Geometry check sheet. Reference: the model listing, model coordinates, mm. Coordinates: 2 decimals unless noted, no trailing zeros. Write each loop counter-clockwise with the first axis right and the second up, starting at its lowest first coordinate (ties: lowest second). Pieces come first, ordered by that corner, then holes. Notation, with made-up numbers: (83.25, 19.25) -> (104.25, 19.25) arc R21 ccw to (104.25, 23.25) -> close; hole circle Ø2 at (77.25, 71). An arc over 180 degrees is marked (long way). Use a Markdown table: item, result.
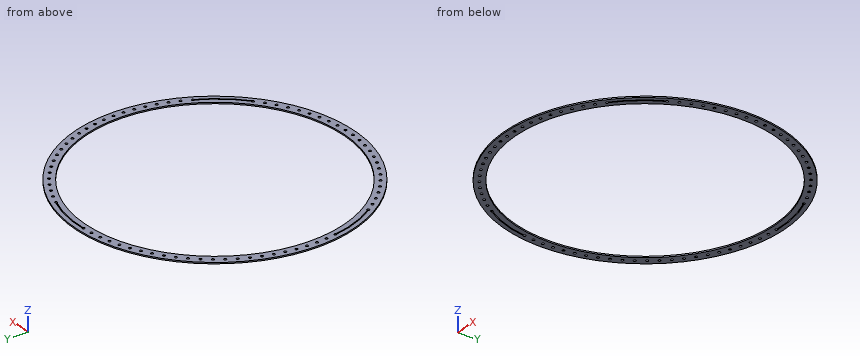
```python
from build123d import *

# Parameters (mm, degrees)
F0_R     = 685.8
F0_R_2   = 6.35
F0_R_3   = 635
F1_DEPTH = 6.35


with BuildPart() as f1:
    # F0 (on Top) → F1 (new body)
    with BuildSketch(Plane.XY):
        Circle(F0_R)
        with Locations((-352.110822, -558.700393)):
            Circle(F0_R_2, mode=Mode.SUBTRACT)
        with Locations((-393.085485, -530.671237)):
            Circle(F0_R_2, mode=Mode.SUBTRACT)
        with Locations((-532.658582, -390.388261)):
            Circle(F0_R_2, mode=Mode.SUBTRACT)
        with Locations((-431.838824, -499.643263)):
            Circle(F0_R_2, mode=Mode.SUBTRACT)
        with Locations((-501.827608, -429.298511)):
            Circle(F0_R_2, mode=Mode.SUBTRACT)
        with Locations((-468.16081, -465.782799)):
            Circle(F0_R_2, mode=Mode.SUBTRACT)
        with Locations((-264.434964, -605.146519)):
            Circle(F0_R_2, mode=Mode.SUBTRACT)
        with Locations((-218.229223, -623.301024)):
            Circle(F0_R_2, mode=Mode.SUBTRACT)
        with Locations((-309.146385, -583.572337)):
            Circle(F0_R_2, mode=Mode.SUBTRACT)
        with Locations((-122.386184, -648.96054)):
            Circle(F0_R_2, mode=Mode.SUBTRACT)
        with Locations((-170.79027, -637.933259)):
            Circle(F0_R_2, mode=Mode.SUBTRACT)
        with Locations((-73.290494, -656.320549)):
            Circle(F0_R_2, mode=Mode.SUBTRACT)
        with Locations((-23.78064, -659.971697)):
            Circle(F0_R_2, mode=Mode.SUBTRACT)
        with BuildLine():
            ThreePointArc((-561.930553, -343.089944), (-556.535629, -344.295153), (-554.129507, -349.271931))
            ThreePointArc((-554.129507, -349.271931), (-562.262715, -355.36641), (-565.827987, -345.849027))
            Line((-565.827987, -345.849027), (-601.958696, -284.23674))
            Line((-601.958696, -284.23674), (-634.753594, -200.992062))
            Line((-634.753594, -200.992062), (-649.807483, -131.860068))
            ThreePointArc((-649.807483, -131.860068), (-652.263014, -120.699131), (-641.979851, -125.684382))
            ThreePointArc((-641.979851, -125.684382), (-642.840203, -128.875975), (-645.188124, -131.202719))
            Line((-645.188124, -131.202719), (-630.639189, -198.568385))
            Line((-630.639189, -198.568385), (-598.505303, -280.938769))
            Line((-598.505303, -280.938769), (-561.930553, -343.089944))
        make_face(mode=Mode.SUBTRACT)
        with Locations((-655.939404, -76.62675)):
            Circle(F0_R_2, mode=Mode.SUBTRACT)
        with Locations((-659.842248, -27.136101)):
            Circle(F0_R_2, mode=Mode.SUBTRACT)
        with Locations((25.863599, -659.893351)):
            Circle(F0_R_2, mode=Mode.SUBTRACT)
        with Locations((75.361682, -656.085952)):
            Circle(F0_R_2, mode=Mode.SUBTRACT)
        with Locations((124.433897, -648.571018)):
            Circle(F0_R_2, mode=Mode.SUBTRACT)
        with Locations((172.802937, -637.391014)):
            Circle(F0_R_2, mode=Mode.SUBTRACT)
        with Locations((220.195469, -622.609119)):
            Circle(F0_R_2, mode=Mode.SUBTRACT)
        with Locations((266.343678, -604.308866)):
            Circle(F0_R_2, mode=Mode.SUBTRACT)
        with Locations((310.986782, -582.593667)):
            Circle(F0_R_2, mode=Mode.SUBTRACT)
        with Locations((353.872502, -557.586238)):
            Circle(F0_R_2, mode=Mode.SUBTRACT)
        with Locations((394.758491, -529.427893)):
            Circle(F0_R_2, mode=Mode.SUBTRACT)
        with BuildLine():
            ThreePointArc((578.330809, -315.516767), (580.121908, -305.046288), (589.006867, -310.868357))
            ThreePointArc((589.006867, -310.868357), (587.146995, -315.358485), (582.656867, -317.218357))
            Line((582.656867, -317.218357), (547.185732, -379.019656))
            Line((547.185732, -379.019656), (491.732303, -449.04348))
            Line((491.732303, -449.04348), (439.763704, -498.277755))
            ThreePointArc((439.763704, -498.277755), (427.529669, -500.665355), (437.968229, -493.852961))
            Line((437.968229, -493.852961), (487.90386, -446.189437))
            Line((487.90386, -446.189437), (542.557285, -377.844919))
            Line((542.557285, -377.844919), (578.330809, -315.516767))
        make_face(mode=Mode.SUBTRACT)
        with Locations((604.36299, -266.220841)):
            Circle(F0_R_2, mode=Mode.SUBTRACT)
        with Locations((622.653864, -220.068912)):
            Circle(F0_R_2, mode=Mode.SUBTRACT)
        with Locations((637.361585, -172.911452)):
            Circle(F0_R_2, mode=Mode.SUBTRACT)
        with Locations((648.549823, -124.544316)):
            Circle(F0_R_2, mode=Mode.SUBTRACT)
        with Locations((656.073112, -75.473382)):
            Circle(F0_R_2, mode=Mode.SUBTRACT)
        with Locations((659.888938, -25.975947)):
            Circle(F0_R_2, mode=Mode.SUBTRACT)
        with Locations((-660.016329, 22.507894)):
            Circle(F0_R_2, mode=Mode.SUBTRACT)
        with Locations((-656.460664, 72.024697)):
            Circle(F0_R_2, mode=Mode.SUBTRACT)
        with Locations((-649.195345, 121.134488)):
            Circle(F0_R_2, mode=Mode.SUBTRACT)
        with Locations((-638.261428, 169.55975)):
            Circle(F0_R_2, mode=Mode.SUBTRACT)
        with Locations((-623.720702, 217.026832)):
            Circle(F0_R_2, mode=Mode.SUBTRACT)
        with Locations((-605.655336, 263.267496)):
            Circle(F0_R_2, mode=Mode.SUBTRACT)
        with Locations((-584.167416, 308.020438)):
            Circle(F0_R_2, mode=Mode.SUBTRACT)
        with Locations((-559.378371, 351.032759)):
            Circle(F0_R_2, mode=Mode.SUBTRACT)
        with Locations((-531.428284, 392.061398)):
            Circle(F0_R_2, mode=Mode.SUBTRACT)
        with Locations((-500.4751, 430.8745)):
            Circle(F0_R_2, mode=Mode.SUBTRACT)
        with Locations((-466.693735, 467.252734)):
            Circle(F0_R_2, mode=Mode.SUBTRACT)
        with Locations((-430.275088, 500.990527)):
            Circle(F0_R_2, mode=Mode.SUBTRACT)
        with Locations((-391.42496, 531.897227)):
            Circle(F0_R_2, mode=Mode.SUBTRACT)
        with Locations((-350.362894, 559.79818)):
            Circle(F0_R_2, mode=Mode.SUBTRACT)
        with Locations((-307.320929, 584.535719)):
            Circle(F0_R_2, mode=Mode.SUBTRACT)
        with Locations((-262.542296, 605.970051)):
            Circle(F0_R_2, mode=Mode.SUBTRACT)
        with Locations((-216.28004, 623.980051)):
            Circle(F0_R_2, mode=Mode.SUBTRACT)
        with Locations((-168.795586, 638.463946)):
            Circle(F0_R_2, mode=Mode.SUBTRACT)
        with Locations((-120.35727, 649.339886)):
            Circle(F0_R_2, mode=Mode.SUBTRACT)
        with Locations((-71.238816, 656.546412)):
            Circle(F0_R_2, mode=Mode.SUBTRACT)
        Circle(F0_R_3, mode=Mode.SUBTRACT)
        with Locations((659.975736, 23.668277)):
            Circle(F0_R_2, mode=Mode.SUBTRACT)
        with Locations((656.333018, 73.178752)):
            Circle(F0_R_2, mode=Mode.SUBTRACT)
        with Locations((648.981367, 122.275694)):
            Circle(F0_R_2, mode=Mode.SUBTRACT)
        with Locations((637.962328, 170.681658)):
            Circle(F0_R_2, mode=Mode.SUBTRACT)
        with Locations((623.338169, 218.1231)):
            Circle(F0_R_2, mode=Mode.SUBTRACT)
        with Locations((583.624962, 309.047025)):
            Circle(F0_R_2, mode=Mode.SUBTRACT)
        with Locations((605.191532, 264.331932)):
            Circle(F0_R_2, mode=Mode.SUBTRACT)
        with BuildLine():
            ThreePointArc((-15.43927, 659.09272), (-27.892825, 658.562438), (-16.552502, 663.736345))
            Line((-16.552502, 663.736345), (53.381546, 663.736345))
            Line((53.381546, 663.736345), (144.287124, 649.791609))
            Line((144.287124, 649.791609), (210.526942, 628.677552))
            ThreePointArc((210.526942, 628.677552), (217.501997, 630.270613), (221.532645, 624.359343))
            ThreePointArc((221.532645, 624.359343), (215.256126, 618.009768), (208.834346, 624.212392))
            Line((208.834346, 624.212392), (139.948994, 646.180678))
            Line((139.948994, 646.180678), (52.268314, 659.09272))
            Line((52.268314, 659.09272), (-15.43927, 659.09272))
        make_face(mode=Mode.SUBTRACT)
        with Locations((306.292743, 585.075136)):
            Circle(F0_R_2, mode=Mode.SUBTRACT)
        with Locations((261.476495, 606.430707)):
            Circle(F0_R_2, mode=Mode.SUBTRACT)
        with Locations((465.871506, 468.072537)):
            Circle(F0_R_2, mode=Mode.SUBTRACT)
        with Locations((499.716777, 431.753752)):
            Circle(F0_R_2, mode=Mode.SUBTRACT)
        with Locations((429.393599, 501.746248)):
            Circle(F0_R_2, mode=Mode.SUBTRACT)
        with Locations((558.760333, 352.015697)):
            Circle(F0_R_2, mode=Mode.SUBTRACT)
        with Locations((530.738153, 392.99513)):
            Circle(F0_R_2, mode=Mode.SUBTRACT)
        with Locations((390.489192, 532.584595)):
            Circle(F0_R_2, mode=Mode.SUBTRACT)
        with Locations((349.378134, 560.413311)):
            Circle(F0_R_2, mode=Mode.SUBTRACT)
    extrude(amount=F1_DEPTH)


solid = f1.part
```
Item 1: Depth check by flat-ended pin: P1, Ø3, axis at x = 408, z = 3.5, coming from the -Y side; P2, Ø1, axis at y = 294.5, z = 1.5, coming from the +X side; P3, Ø10, axis at x = -560.48, y = -349.27, coming from the -Z side; P4, Ø1, axis at x = 178, z = 1.5, coming from the -Y side. Enter the tip coordinate at first touch or a pass-through.
Answer block:
| item | result |
|---|---|
| P1 | stops at y = -552.34 |
| P2 | stops at x = 619.59 |
| P3 | passes through |
| P4 | stops at y = -662.43 |
Item 2: Section check B-B on z = 5. Count the separate pieces of the cut face and the enclosed holes in it, then the cut area to 3 significant figures.
Answer block:
| item | result |
|---|---|
| separate pieces | 1 |
| enclosed holes | 70 |
| area | 198,000 mm^2 |
Item 3: Section check A-A on y = 0. Record the boundary of the cut face in (x, z).
Answer block:
| item | result |
|---|---|
| outline | (-685.8, 0) -> (-635, 0) -> (-635, 6.35) -> (-685.8, 6.35) -> close; (635, 0) -> (685.8, 0) -> (685.8, 6.35) -> (635, 6.35) -> close |
Item 4: Thickness scan on L1, parallel to Y at x = 216.5, z = 6.25; L2, parallel to Y at x = 427, z = 3; L3, parallel to X at y = -176.5, z = 1.75. Record the ranges inside material, lowest first. Write a range as [from, to].
Answer block:
| item | result |
|---|---|
| L1 | y = [-650.73, -627.77], [-617.45, -596.95], [596.95, 618.15], [630.57, 650.73] |
| L2 | y = [-536.65, -470], [470, 495.86], [507.63, 536.65] |
| L3 | x = [-662.7, -640.09], [-635.41, -609.98], [609.98, 632.12], [642.6, 662.7] |
